```python
from build123d import *

# Parameters (mm, degrees)
SKETCH_1_R          = 12.5
EXTRUDE_1_DEPTH     = 35
SKETCH_3_W          = 7
SKETCH_3_H          = 3
EXTRUDE_2_DEPTH     = 5
SKETCH_4_R          = 1.5
CUT_EXTRUDE_1_DEPTH = 5
FILLET_1_R          = 3
FILLET_2_R          = 3
FILLET_3_R          = 7
SKETCH_5_R          = 7
CUT_EXTRUDE_2_DEPTH = 30


with BuildPart() as part:
    # 草图1 → 凸台-拉伸1 (new body)
    with BuildSketch(Plane(origin=(0, 0, 0), x_dir=(0, 0, -1), z_dir=(1, 0, 0))):
        Circle(SKETCH_1_R)
    extrude(amount=-EXTRUDE_1_DEPTH)

    # 草图3 → 凸台-拉伸2 (add)
    with BuildSketch(Plane.ZY.offset(35)):
        Rectangle(SKETCH_3_W, SKETCH_3_H)
    extrude(amount=EXTRUDE_2_DEPTH)

    # 草图4 → 切除-拉伸1 (cut)
    with BuildSketch(Plane.XZ.offset(1.5)):
        with Locations(Location((-37.5, 0, 0), (0, 0, 270))):
            Circle(SKETCH_4_R)
    extrude(amount=-CUT_EXTRUDE_1_DEPTH, mode=Mode.SUBTRACT)

    # 圆角1
    fillet_1_edges = [part.edges().sort_by_distance(p)[0] for p in [
        (-40, 0, 3.5),
    ]]
    fillet(fillet_1_edges, radius=FILLET_1_R)

    # 圆角2
    fillet_2_edges = [part.edges().sort_by_distance(p)[0] for p in [
        (-40, 0, -3.5),
    ]]
    fillet(fillet_2_edges, radius=FILLET_2_R)

    # 圆角3
    fillet_3_edges = [part.edges().sort_by_distance(p)[0] for p in [
        (-35, 0, 12.5),
    ]]
    fillet(fillet_3_edges, radius=FILLET_3_R)

    # 草图5 → 切除-拉伸2 (cut)
    with BuildSketch(Plane(origin=(0, 0, 0), x_dir=(0, 0, -1), z_dir=(1, 0, 0))):
        Circle(SKETCH_5_R)
    extrude(amount=-CUT_EXTRUDE_2_DEPTH, mode=Mode.SUBTRACT)


solid = part.part
```
Source: CAD feature listing. Evaluate the final solid. Frame: model axes, mm. A direction names the side the tool comes from. Coordinates: 2 decimals unless noted, no trailing zeros. Write each loop counter-clockwise with the first axis right and the second up, starting at its lowest first coordinate (ties: lowest second). Pieces come first, ordered by that corner, then holes. Notation, with made-up numbers: (79.5, 58) -> (130.5, 58) arc R12 cw to (130.5, 77) -> close; hole circle Ø1 at (-30, -34). An arc over 180 degrees is marked (long way). Return JSON: item names as keys, results as strings. Group by question number.
1) Ray query, line 1 along X through (y, z) = (-0.75, 0); line 2 along X through (y, z) = (-2.25, 0.5); line 3 along Z through (x, y) = (-22.5, -2). Return the intervals inside material, ascending.
2) Section query B-B, the plane x = -26. Return loops of the section in (y, z).
3) Mould query, pull axis Y, two halves, no side actions, for faces 4 (the face through (-13.804, 3.755, -11.923)), 5 (the face through (-36, 0, -3.5)), 6 (the face through (-30, 0, 0)). Classes: +Y half, -Y half, draft (parallel to the pull), parting line (faces both ways), or undercut.
4) Contact query for flat-ended pins moving along their axis: P1, Ø6, axis at x = -14, y = -2, coming from the +Z side; P2, Ø7, axis at y = -0.5, z = -1.5, coming from the +X side; P3, Ø4, axis at x = -34, z = -6.5, coming from the -Y side; P4, Ø1, axis at x = -36, y = 0, coming from the -Z side. Output: stop coordinate, or through.
5) Set-up query: faces 1 (the face through (-35.8, -1.5, 0)), 2 (the face through (-36, 0, 3.5)), 3 (the face through (-14.79, -2.681, -6.466)). Return all of +Z, -Z, +X, -X, +Y, -Y with unobstructed straight access to the full face (end or side cutting, diameter ignored); none if empty.
6) Section query A-A, the plane x = -37.5. Return loops of the section in (y, z).
From the geometry:
{
 "1": {"line 1": "-40 to -39, -36 to -30", "line 2": "-35 to -30", "line 3": "-12.34 to -6.71, 6.71 to 12.34"},
 "2": {"outline": "circle Ø25 at (0, 0); hole circle Ø14 at (0, 0)"},
 "3": {"face 4": "parting line", "face 5": "draft", "face 6": "undercut"},
 "4": {"P1": "z = 12.5", "P2": "x = -30", "P3": "y = -9.58", "P4": "z = -3.5"},
 "5": {"face 1": "+Z, -Z, -X, -Y", "face 2": "+Z, -X, +Y, -Y", "face 3": "+X"},
 "6": {"outline": "(-1.5, -3.46) -> (1.5, -3.46) -> (1.5, -1.5) -> (-1.5, -1.5) -> close; (-1.5, 1.5) -> (1.5, 1.5) -> (1.5, 3.46) -> (-1.5, 3.46) -> close"}
}
